Design review of the part built by this model. Coordinates are the model's own, in mm. A direction names the side the tool comes from. Round coordinates to 2 decimals unless told otherwise and drop trailing zeros. Order: outer loops, then holes, each group sorted by start corner. A loop starts at its lowest first (then second) coordinate and runs counter-clockwise, first axis right, second up.
from build123d import *

# Parameters (mm, degrees)
F0_R     = 4
F0_R_2   = 2.5
F1_DEPTH = 12
F2_R     = 3
F2_R_2   = 2.5
F3_DEPTH = 5
F4_SIZE2 = 0.99999
F4_SIZE  = 2.99999


# Not quite as in the source:
# - a fillet or chamfer is up to 0.001 mm smaller than in the source, because OpenCascade refuses the exact size


with BuildPart() as f1:
    # F0 (on Front) → F1 (new body)
    with BuildSketch(Plane.XZ):
        Circle(F0_R)
        Circle(F0_R_2, mode=Mode.SUBTRACT)
    extrude(amount=F1_DEPTH)

    # F2 (on face) → F3 (join)
    with BuildSketch(Plane(origin=(0, 0, 0), x_dir=(-1, 0, 0), z_dir=(0, 1, 0))):
        Circle(F2_R)
        Circle(F2_R_2, mode=Mode.SUBTRACT)
    extrude(amount=F3_DEPTH)

    # F4 (size 3 and 1 in the source; OpenCascade refuses exactly that, so slightly less here)
    f4_edges = [f1.edges().sort_by_distance(p)[0] for p in [
        (-4, 0, 0),
    ]]
    f4_side = f1.faces().sort_by_distance((-4, -6, 0))[0]
    chamfer(f4_edges, length=F4_SIZE, length2=F4_SIZE2, reference=f4_side)


solid = f1.part
1) To check wall thickness, follow line 1 along Z through (x, y) = (0, -8); line 2 along Z through (x, y) = (0, 3.35); line 3 along X through (y, z) = (-11, -0.75). State the ranges of each line that lie inside material, in increasing order.
Results:
line 1: z = -4 to -2.5, 2.5 to 4
line 2: z = -3 to -2.5, 2.5 to 3
line 3: x = -3.93 to -2.38, 2.38 to 3.93
2) Clearance check with flat-ended pins moving along their axes: P1, Ø3, axis at x = -2.5, y = -2, coming from the +Z side; P2, Ø4, axis at x = -2, y = 2.5, coming from the -Z side; P3, Ø4, axis at y = 2.5, z = 2, coming from the -X side. State where each tip first meets the part, or that it passes through.
Results:
P1: stops at z = 3.75
P2: stops at z = -3
P3: stops at x = -3
3) Take a section at C-C on y = 1. Give the boundary of the cut face in (x, z).
Results:
outline: circle Ø6 at (0, 0); hole circle Ø5 at (0, 0)
4) For faces 1 (the face through (3, 2, 0)), 2 (the face through (2, -12, 2)), list the 3-axis set-ups (+Z, -Z, +X, -X, +Y, -Y) from which the entire face can be reached by the end or side of a thin tool; tool diameter is ignored.
Results:
face 1: +Y
face 2: +Z, -Z, +X, -X, -Y
5) Take a section at D-D on y = -3.75. Give the boundary of the cut face in (x, z), plus the area to 3 significant figures.
Results:
outline: circle Ø8 at (0, 0); hole circle Ø5 at (0, 0)
area: 30.6 mm2
